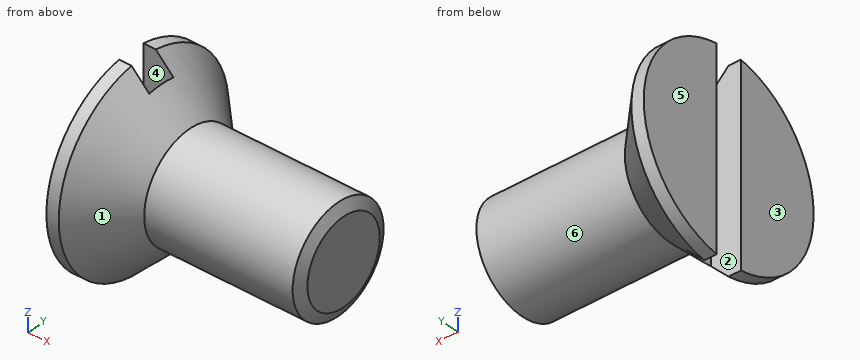
Autodesk Inventor part; units mm, degrees
ref_plane "Work Plane1" through (33.575, 0, 0) normal (0, 0, -1) x (1, 0, 0)
ref_plane "YZ Plane" through (0, 0, 0) normal (1, 0, 0) x (0, 1, 0)
ref_plane "XZ Plane" through (0, 0, 0) normal (0, 1, 0) x (-1, 0, 0)
sketch "Skizze1" plane through (0, 0, 0) normal (0, 0, 1) x (1, 0, 0)
  line L0 (0, 0) -> (6, 0)
  line L1 (6, 0) -> (6, 1.5)
  line L2 (6, 1.5) -> (2.65, 1.5)
  line L3 (2.65, 1.5) -> (2.3433, 1.5)
  line L4 (2.3433, 1.5) -> (1.65, 1.5)
  line L5 (1.65, 1.5) -> (0.35, 2.8)
  line L6 (0.35, 2.8) -> (0, 2.8)
  line L7 (0, 2.8) -> (0, 0)
  line L8 (2.65, 1.5) -> (1.65, 1.5) construction
  line L9 (-1.2, 0) -> (7.2, 0)
  line L10 (0, 3.36) -> (0, -0.56)
  dimension "d0" = 6
  dimension "d1" = 45
  dimension "d2" = 0.3067
  dimension "d3" = 3.35
  dimension "d4" = 1.65
  dimension "d5" = 3
  dimension "d6" = 3
  dimension "d7" = 5.6
revolve "Körper" add sketch "Skizze1" angle 360 about axis through (0, 0, 0) along (1, 0, 0)
sketch "Skizze2" plane through (0, 0, 0) normal (-1, 0, 0) x (0, 0, 1)
  line L0 (2.8, -0.4) -> (-2.8, -0.4)
  line L1 (-2.8, -0.4) -> (-2.8, 0.4)
  line L2 (-2.8, 0.4) -> (2.8, 0.4)
  line L3 (2.8, 0.4) -> (2.8, -0.4)
  line L4 (0, 0.4) -> (0, -0.4) construction
  line L5 (-2.8, 0) -> (2.8, 0) construction
  line L6 (0, 2.8) -> (0, 0)
  dimension "d15" = 0.8
  dimension "d16" = 5.6
extrude "Loch" cut sketch "Skizze2" against normal blind 0.85
thread "Gewinde"
chamfer "Fase1" distance 0.3067 distance2 0.1534 1 edges at (6, -1.5, 0) measured on face at (6, -0.5112, 0.3316)
ref_plane "Work Plane1" through (33.575, 0, 0) normal (0, 0, -1) x (1, 0, 0)
equation "\"d1\" = 0.5 * SEWI"
equation "\"d2\" = GAL"
equation "\"d4\" = KOH"
equation "\"d5\" = BDM"
equation "\"d6\" = GD"
equation "\"d7\" = KOD"
equation "\"d15\" = SBR"
equation "\"d16\" = KOD"
equation "\"d8\" = STI"
equation "\"d12\" = -0.5 * SPD + 0.5 * GD"
equation "\"d13\" = 0.5 * GAL"
equation "\"NLG\" = 4"
equation "\"GAL\" = 0.61345 * PTC"
equation "\"GEL\" = 1.35"
equation "\"KOH\" = 1.65"
equation "\"KOD\" = 5.6"
equation "\"SEWI\" = 90deg"
equation "\"BDM\" = NND"
equation "\"GD\" = NND"
equation "\"SBR\" = 0.8"
equation "\"STI\" = 0.85"
equation "\"SPD\" = NND - 1.2269 * PTC"
equation "\"GUL\" = 0.61345 * PTC"
equation "\"PTC\" = 0.5"
equation "\"EPV\" = 3.15"
equation "\"THREADDIA\" = 3"
equation "\"TOA\" = 30deg"
equation "\"NND\" = 3"
equation "\"GD1\" = THREADDIA - 1.2269 * PTC"
properties part number "DIN 963 - M3 x 4" material "Edelstahl"
Can you work these out from the model? Positions are in its coordinate system, mm. Face numbers are marked on the shaded views. A direction names the side the tool comes from. Coordinates: 2 decimals unless noted, no trailing zeros. Order: outer loops, then holes, each group sorted by start corner. A loop starts at its lowest first (then second) coordinate and runs counter-clockwise, first axis right, second up. Notation, with made-up numbers: (33.25, 33) - (54.25, 33) arc R33 cw to (54.25, 63) - close; hole circle Ø9 at (28.5, 22.5). An arc over 180 degrees is marked (long way). Answer in a Markdown table with one row per item.
1. For pin 1 (2 mm diameter, centred on x = 5, y = -2, fed in from -Z); pin 2 (0.6 mm diameter, centred on y = 0, z = 0.5, fed in from -X); pin 3 (1.5 mm diameter, centred on x = 3.5, z = 0, fed in from -Y), each with a flat end and sliding along its axis, tell me the tip position at first contact or that it passes through.
Reply:
| item | result |
|---|---|
| pin 1 | stops at z = -1.12 |
| pin 2 | stops at x = 0.85 |
| pin 3 | stops at y = -1.5 |
2. Suppose I cut it at C-C (x = 5.5). Please give me the cut outline in (y, z).
Reply:
| item | result |
|---|---|
| outline | circle Ø3 at (0, 0) |
3. If we mould it in two halves opening along Y, with no side actions, what happens to the marked faces 1, 2, 3 and 4? For each: pulls with the +Y half, pulls with the -Y half, needs draft (parallel to the pull), parting line crosses it, or undercut.
Reply:
| item | result |
|---|---|
| face 1 | parting line crosses it |
| face 2 | undercut |
| face 3 | needs draft |
| face 4 | undercut |
4. Suppose I cut it at B-B (y = 0). Please give me the cut outline in (x, z).
Reply:
| item | result |
|---|---|
| outline | (0.85, -2.3) - (1.65, -1.5) - (5.85, -1.5) - (6, -1.19) - (6, 1.19) - (5.85, 1.5) - (1.65, 1.5) - (0.85, 2.3) - close |
5. If I drill on line 1 along X through (y, z) = (-0.9, -2.15); line 2 along Y through (x, z) = (3, -0.75); line 3 along Y through (x, z) = (0.5, -0.1), over which ranges is the centre line in solid material (lowest first)?
Reply:
| item | result |
|---|---|
| line 1 | x = 0 to 0.82 |
| line 2 | y = -1.3 to 1.3 |
| line 3 | y = -2.65 to -0.4, 0.4 to 2.65 |
6. For the marked faces 5 and 6, which set-ups out of +Z, -Z, +X, -X, +Y, -Y let a thin tool reach every point of the face, with its end or its side?
Reply:
| item | result |
|---|---|
| face 5 | +Z, -Z, -X, +Y, -Y |
| face 6 | +X |
7. Suppose I cut it at D-D (x = 1.5). Please give me the cut outline in (y, z), and give its area (3 significant figures).
Reply:
| item | result |
|---|---|
| outline | circle Ø3.3 at (0, 0) |
| area | 8.55 mm^2 |
8. Suppose I cut it at A-A (z = 0). Please give me the cut outline in (x, y), and give its area (3 significant figures).
Reply:
| item | result |
|---|---|
| outline | (0, -2.8) - (0.35, -2.8) - (1.65, -1.5) - (5.85, -1.5) - (6, -1.19) - (6, 1.19) - (5.85, 1.5) - (1.65, 1.5) - (0.35, 2.8) - (0, 2.8) - (0, 0.4) - (0.85, 0.4) - (0.85, -0.4) - (0, -0.4) - close |
| area | 19.9 mm^2 |
